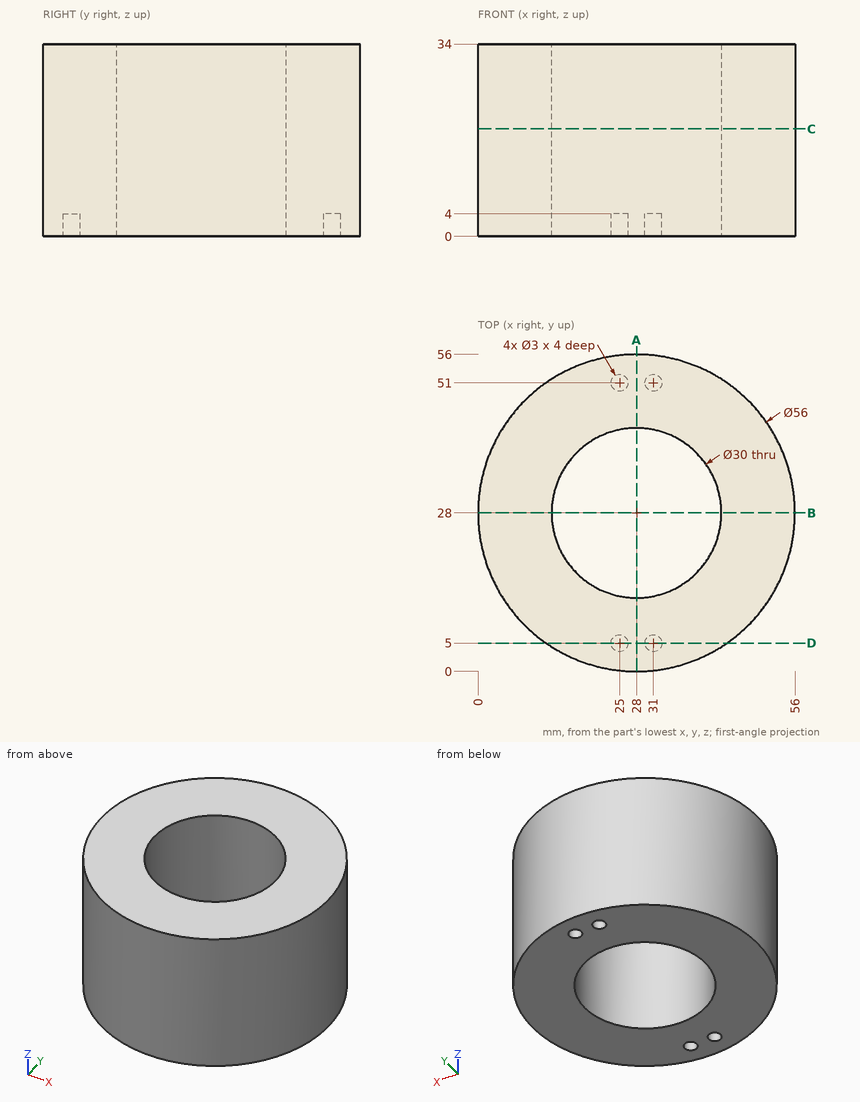
The figure shows three views and two pictorial views of one solid part (mm, origin at its lowest corner). Answer the questions. Give positions to 0.01 mm unless a question says otherwise; leave off trailing zeros. Write each loop counter-clockwise with the first axis right and the second up, starting at its lowest first coordinate (ties: lowest second). Pieces come first, ordered by that corner, then holes. Notation, with made-up numbers: (-5.5, 69) - (25.5, 69) arc R27 cw to (25.5, 106) - close; hole circle Ø11 at (-8.5, 7). An arc over 180 degrees is marked (long way). Use one line per item in the form item = value.
1. A cutting plane is placed at D-D (y = 5). Write down the section's boundary in (x, z), and give its area (3 significant figures).
Filled in:
outline = (12.03, 0) - (23.5, 0) - (23.5, 4) - (26.5, 4) - (26.5, 0) - (29.5, 0) - (29.5, 4) - (32.5, 4) - (32.5, 0) - (43.97, 0) - (43.97, 34) - (12.03, 34) - close
area = 1,060 mm^2
2. A cutting plane is placed at A-A (x = 28). Write down the section's boundary in (y, z), and give its area (3 significant figures).
Filled in:
outline = (0, 0) - (13, 0) - (13, 34) - (0, 34) - close; (43, 0) - (56, 0) - (56, 34) - (43, 34) - close
area = 884 mm^2
3. Each of these flat-tipped pins is pushed along its axis until it touches: pin 1 Ø3 at (x, z) = (10, 13.5) entering from +Y; pin 2 Ø1.8 at (x, y) = (31, 51) entering from -Z; pin 3 Ø10 at (y, z) = (50, 7.5) entering from -X. Where does it stop, or does it pass through?
Filled in:
pin_1 = 50.62
pin_2 = 4
pin_3 = 5.75
4. A cutting plane is placed at C-C (z = 19). Write down the section's boundary in (x, y), and give its area (3 significant figures).
Filled in:
outline = circle Ø56 at (28, 28); hole circle Ø30 at (28, 28)
area = 1,760 mm^2
5. Consider L1, parallel to Y at x = 25, z = 2.85; L2, parallel to X at y = 5, z = 1.45; L3, parallel to X at y = 23.5, z = 13. Determine where each line is inside the solid, lowest interval first.
Filled in:
L1 = 0.16 to 3.5, 6.5 to 13.3, 42.7 to 49.5, 52.5 to 55.84
L2 = 12.03 to 23.5, 26.5 to 29.5, 32.5 to 43.97
L3 = 0.36 to 13.69, 42.31 to 55.64
